For this review, take the finished solid that the model builds, in its own axes (mm). Face numbers are marked on the shaded views. A direction names the side the tool comes from. Coordinates: 2 decimals unless noted, no trailing zeros. Write each loop counter-clockwise with the first axis right and the second up, starting at its lowest first coordinate (ties: lowest second). Pieces come first, ordered by that corner, then holes. Notation, with made-up numbers: (74, 55) - (115, 55) arc R7 cw to (115, 59) - close; hole circle Ø5 at (52, 59.5). An arc over 180 degrees is marked (long way). Use one line per item in the form item = value. Start each with the question number.
1) Insertion check: P1, Ø0.9, axis at x = -30, z = 7.5, coming from the +Y side; P2, Ø10, axis at x = -34, y = -3, coming from the +Z side; P3, Ø1.5, axis at x = -28, z = 7.5, coming from the -Y side; P4, Ø6, axis at y = -9, z = 5, coming from the -X side. Each pin has a flat end and moves straight along its axis. Give the tip position at first contact, or say it passes through.
2) For L1, parallel to Y at x = 0, z = 3.5; L2, parallel to X at y = -12.5, z = 7.25; L3, parallel to Y at x = 4.5, z = 11.5, list the stretches that pass through material, from the lowest coordinate up. Write a range as from..to.
3) We need section B-B (x = 0). Give the boundary of the cut face in (y, z).
4) We need section C-C (z = 2.75). Give the boundary of the cut face in (x, y), plus the area to 3 significant figures.
5) We need section D-D (y = -7). Give the boundary of the cut face in (x, z), plus the area to 3 significant figures.
6) We need section A-A (y = 0). Give the boundary of the cut face in (x, z), plus the area to 3 significant figures.
7) Mouldability with a two-part tool opening along X and no side actions: class the marked faces 4, 5 and 6 as pulls with the +X half, pulls with the -X half, needs draft (parallel to the pull), parting line crosses it, or undercut.
8) Tool access review of the marked faces 1, 2 and 3: name each direction out of +Z, -Z, +X, -X, +Y, -Y from which nothing blocks a thin tool from reaching the whole face with its end or side.
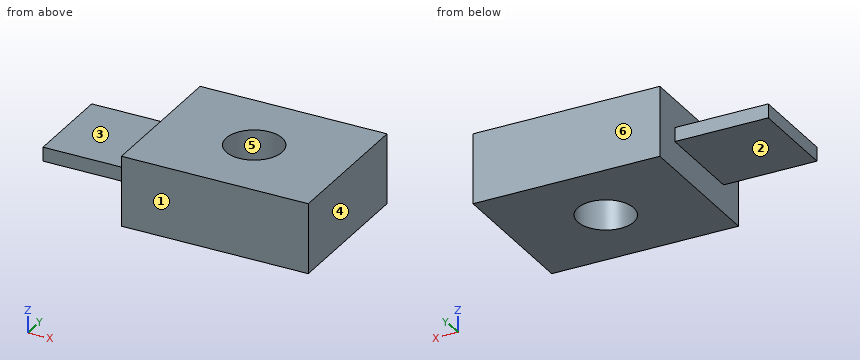
```python
from build123d import *

# Parameters (mm, degrees)
SKETCH1_W           = 40
SKETCH1_H           = 31.5
BOSS_EXTRUDE1_DEPTH = 15
SKETCH2_W           = 3
SKETCH2_H           = 19.5
BOSS_EXTRUDE2_DEPTH = 20
SKETCH3_R           = 6
CUT_EXTRUDE1_DEPTH  = 46.530896104


with BuildPart() as part:
    # Sketch1 → Boss-Extrude1 (new body)
    with BuildSketch(Plane.XY):
        Rectangle(SKETCH1_W, SKETCH1_H)
    extrude(amount=BOSS_EXTRUDE1_DEPTH)

    # Sketch2 → Boss-Extrude2 (add)
    with BuildSketch(Plane.ZY.offset(20)):
        with Locations((7.5, 0)):
            Rectangle(SKETCH2_W, SKETCH2_H)
    extrude(amount=BOSS_EXTRUDE2_DEPTH)

    # Sketch3 → Cut-Extrude1 (cut, through all)
    with BuildSketch(Plane(origin=(0, 0, 0), x_dir=(-1, 0, 0), z_dir=(0, 0, -1))):
        Circle(SKETCH3_R)
    extrude(amount=-CUT_EXTRUDE1_DEPTH, mode=Mode.SUBTRACT)


solid = part.part
```
Determined:
q1.P1 = 9.75
q1.P2 = 9
q1.P3 = -9.75
q1.P4 = -40
q2.L1 = -15.75..-6, 6..15.75
q2.L2 = -20..20
q2.L3 = -15.75..-3.97, 3.97..15.75
q3.outline = (-15.75, 0) - (-6, 0) - (-6, 15) - (-15.75, 15) - close; (6, 0) - (15.75, 0) - (15.75, 15) - (6, 15) - close
q4.outline = (-20, -15.75) - (20, -15.75) - (20, 15.75) - (-20, 15.75) - close; hole circle Ø12 at (0, 0)
q4.area = 1,150 mm²
q5.outline = (-40, 6) - (-20, 6) - (-20, 0) - (20, 0) - (20, 15) - (-20, 15) - (-20, 9) - (-40, 9) - close
q5.area = 660 mm²
q6.outline = (-40, 6) - (-20, 6) - (-20, 0) - (-6, 0) - (-6, 15) - (-20, 15) - (-20, 9) - (-40, 9) - close; (6, 0) - (20, 0) - (20, 15) - (6, 15) - close
q6.area = 480 mm²
q7.face_4 = pulls with the +X half
q7.face_5 = undercut
q7.face_6 = needs draft
q8.face_1 = +Z, -Z, +X, -X, -Y
q8.face_2 = -Z, -X, +Y, -Y
q8.face_3 = +Z, -X, +Y, -Y
